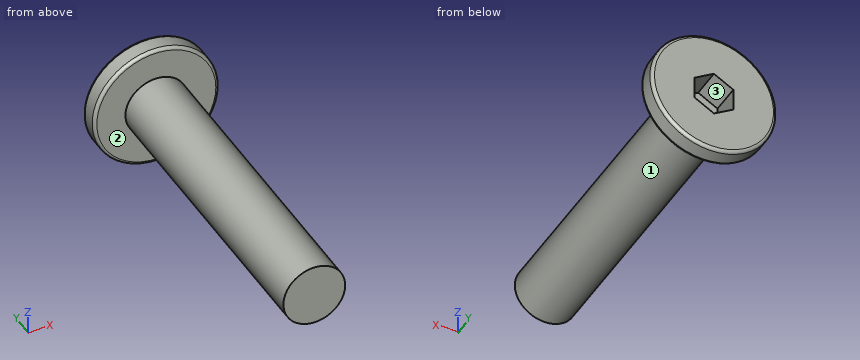
```python
from build123d import *

# Parameters (mm, degrees)
SKETCH1_R           = 4.05
BOSS_EXTRUDE1_DEPTH = 1.3
FILLET1_R           = 0.2
SKETCH2_R           = 2
BOSS_EXTRUDE2_DEPTH = 20
CUT_EXTRUDE1_DEPTH  = 2


with BuildPart() as part:
    # Sketch1 → Boss-Extrude1 (new body)
    with BuildSketch(Plane(origin=(0, 0, 0), x_dir=(1, 0, 0), z_dir=(0, 1, 0))):
        Circle(SKETCH1_R)
    extrude(amount=BOSS_EXTRUDE1_DEPTH)

    # Fillet1
    fillet1_edges = [part.edges().sort_by_distance(p)[0] for p in [
        (-4.05, 0, 0),
        (-4.05, 1.3, 0),
    ]]
    fillet(fillet1_edges, radius=FILLET1_R)

    # Sketch2 → Boss-Extrude2 (add)
    with BuildSketch(Plane.XZ):
        Circle(SKETCH2_R)
    extrude(amount=BOSS_EXTRUDE2_DEPTH)

    # Sketch3 → Cut-Extrude1 (cut)
    with BuildSketch(Plane(origin=(0, 1.3, 0), x_dir=(1, 0, 0), z_dir=(0, 1, 0))):
        Polygon((-1.25, -0.721687836), (0, -1.443375673), (1.25, -0.721687836), (1.25, 0.721687836), (0, 1.443375673), (-1.25, 0.721687836), align=None)
    extrude(amount=-CUT_EXTRUDE1_DEPTH, mode=Mode.SUBTRACT)


solid = part.part
```
Verification items for the finished model (mm, model axes). Face numbers are marked on the shaded views. Round coordinates to 2 decimals unless told otherwise and drop trailing zeros. Loops run counter-clockwise (first coordinate to the right, second up) from the corner with the lowest first, then second, coordinate; pieces in that order, holes last. Notation, with made-up numbers: (-36, -29) -> (-12, -29) arc R10 ccw to (-12, -13) -> close; hole circle Ø9 at (38, 32). An arc over 180 degrees is marked (long way). Answer as a JSON object with one key per item and string values.
Q1. Go/stop test with flat-tipped pins: P1, Ø1, axis at x = -1, y = -3, coming from the +Z side; P2, Ø0.8, axis at x = 0.5, z = -0.5, coming from the +Y side; P3, Ø0.7, axis at y = 0, z = -0.5, coming from the +X side. Record where each tip stops, or that it passes through.
Data:
{"P1": "stops at z = 1.94", "P2": "stops at y = -0.7", "P3": "stops at x = 4.04"}
Q2. Section check A-A (y = -0.5). Record the boundary of the cut face in (x, z).
Data:
{"outline": "circle Ø4 at (0, 0); hole (-1.25, -0.72) -> (0, -1.44) -> (1.25, -0.72) -> (1.25, 0.72) -> (0, 1.44) -> (-1.25, 0.72) -> close"}
Q3. Section check B-B (z = 0). Record the boundary of the cut face in (x, y), then the cut area to 3 significant figures.
Data:
{"outline": "(-4.05, 0.2) arc R0.2 ccw to (-3.85, 0) -> (-2, 0) -> (-2, -20) -> (2, -20) -> (2, 0) -> (3.85, 0) arc R0.2 ccw to (4.05, 0.2) -> (4.05, 1.1) arc R0.2 ccw to (3.85, 1.3) -> (1.25, 1.3) -> (1.25, -0.7) -> (-1.25, -0.7) -> (-1.25, 1.3) -> (-3.85, 1.3) arc R0.2 ccw to (-4.05, 1.1) -> close", "area": "85.5 mm2"}
Q4. Scan lines: line 1 (Y direction, x = -3.5, z = 1.5); line 2 (Y direction, x = -0.75, z = -0.5); line 3 (X direction, y = -16, z = -1.75). Record each from-to range of solid material in increasing order. Write a range as from..to.
Data:
{"line 1": "y = 0..1.3", "line 2": "y = -20..-0.7", "line 3": "x = -0.97..0.97"}
Q5. Draft check along X on the marked faces 1, 2 and 3. Enter one of: pulls with the +X half, pulls with the -X half, needs draft (parallel to the pull), parting line crosses it, or undercut.
Data:
{"face 1": "parting line crosses it", "face 2": "needs draft", "face 3": "undercut"}
Q6. Section check C-C (y = -17.25). Record the boundary of the cut face in (x, z).
Data:
{"outline": "circle Ø4 at (0, 0)"}
